Autodesk Inventor part; units mm, degrees
ref_plane "YZ Plane" through (0, 0, 0) normal (1, 0, 0) x (0, 1, 0)
ref_plane "XZ Plane" through (0, 0, 0) normal (0, 1, 0) x (-1, 0, 0)
ref_plane "XY Plane" through (0, 0, 0) normal (0, 0, 1) x (1, 0, 0)
sketch "Sketch1" plane through (0, 0, 0) normal (0, 0, 1) x (1, 0, 0)
  line L0 (0, 0) -> (-15, 0) construction
  circle A0 centre (-15, 0) radius 4
  line L1 (10, 25) -> (0, 25)
  line L2 (0, 25) -> (0, -25)
  line L3 (0, -25) -> (10, -25)
  line L4 (10, -25) -> (10, 25)
  line L5 (0, 0) -> (-15, 0) construction
  line L6 (0, 7) -> (-15, 7)
  line L7 (-15, -7) -> (0, -7)
  arc A1 (0, -7) -> (0, 7) centre (0, 0) ccw
  arc A2 (-15, 7) -> (-15, -7) centre (-15, 0) ccw
  point P0 (-7.5, 0)
  dimension "d0" = 8
  dimension "d1" = 15
  dimension "d2" = 50
  dimension "d3" = 10
  dimension "d4" = 7
extrude "Extrusion1" add sketch "Sketch1" along normal blind 20
sketch "Sketch2" plane through (10, -25, 0) normal (1, 0, 0) x (0, 0, -1)
  line L0 (0, 50) -> (-20, 50) construction
  line L1 (-10, 50) -> (-10, 40) construction
  line L2 (0, 0) -> (-20, 0) construction
  line L3 (-10, 0) -> (-10, 10) construction
  circle A0 centre (-10, 40) radius 2.5
  circle A1 centre (-10, 10) radius 2.5
  point P0 (0, 25)
  dimension "d7" = 5
  dimension "d8" = 10
extrude "Extrusion2" cut sketch "Sketch2" against normal through all
fillet "Fillet1" radius 6 4 edges at (5, 25, 20) (5, 25, 0) (5, -25, 20) (5, -25, 0)
sketch "Sketch3" plane through (10, -19, 0) normal (1, 0, 0) x (0, 0, -1)
  line L0 (-20, 15) -> (-20, 23)
  line L1 (-20, 19) -> (-30, 19) construction
  line L2 (-20, 26) -> (-30, 26)
  line L3 (-30, 12) -> (-20, 12)
  arc A0 (-20, 12) -> (-20, 26) centre (-20, 19) ccw
  arc A1 (-30, 26) -> (-30, 12) centre (-30, 19) ccw
  circle A2 centre (-30, 19) radius 2.5
  point P0 (0, 19)
  point P1 (-25, 19)
  dimension "d12" = 5
  dimension "d13" = 7
  dimension "d14" = 10
extrude "Extrusion3" add sketch "Sketch3" against normal blind 10
properties part number "frame mount 1"
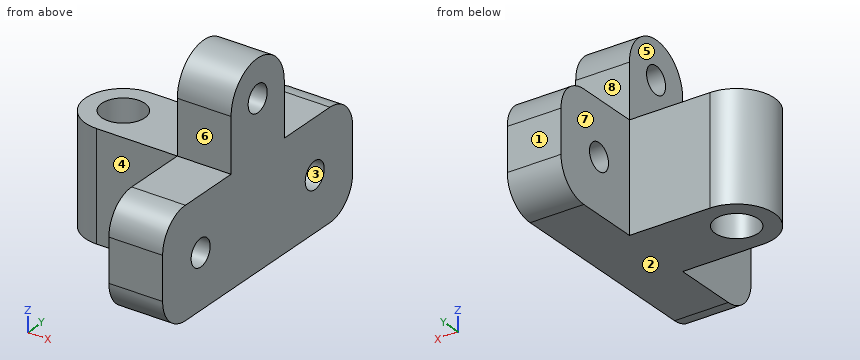
Check sheet for the modelled part. Datum: model origin and axes. Units: mm. Face numbers are marked on the shaded views. A direction names the side the tool comes from. Coordinates: 2 decimals unless noted, no trailing zeros. Write each loop counter-clockwise with the first axis right and the second up, starting at its lowest first coordinate (ties: lowest second). Pieces come first, ordered by that corner, then holes. Notation, with made-up numbers: M -34.5,3.5 L -5.5,3.5 A27 ccw -5.5,19.5 Z; hole C 70,58.25 d6. An arc over 180 degrees is marked long. Use one line per item in the form item = value.
Item 1: Gauge pin test, flat ends, axial feed: pin 1 Ø8 at (x, y) = (-9, -1) entering from +Z; pin 2 Ø7 at (y, z) = (-1, 29) entering from -X; pin 3 Ø14.5 at (y, z) = (-12.5, 8) entering from -X. Record the tip position at first contact, or that the pin passes through.
Answer below:
pin_1 = 20
pin_2 = 0
pin_3 = -19.63
Item 2: Sectioned sample at B-B, the plane z = 10. Record the cut outline in (x, y), and give its area (3 significant figures).
Answer below:
outline = M -15,-7 L 0,-7 L 0,-12.5 L 10,-12.5 L 10,12.5 L 0,12.5 L 0,7 L -15,7 A7 ccw Z; M 0,-25 L 10,-25 L 10,-17.5 L 0,-17.5 Z; M 0,17.5 L 10,17.5 L 10,25 L 0,25 Z; hole C -15,0 d8
area = 637 mm^2
Item 3: Release check for a two-part mould opening along Y. For the marked faces 1, 2 and 3 record: pulls with the +Y half, pulls with the -Y half, needs draft (parallel to the pull), parting line crosses it, or undercut.
Answer below:
face_1 = pulls with the +Y half
face_2 = needs draft
face_3 = undercut
Item 4: Material ranges on L1, parallel to Y at x = 4, z = 10; L2, parallel to Y at x = -15, z = 8.5; L3, parallel to X at y = 2, z = 22.5, recorded low to high. Write a range as from..to.
Answer below:
L1 = -25..-17.5, -12.5..12.5, 17.5..25
L2 = -7..-4, 4..7
L3 = 0..10
Item 5: Sectioned sample at D-D, the plane y = 0. Record the cut outline in (x, z).
Answer below:
outline = M -22,0 L -19,0 L -19,20 L -22,20 Z; M -11,0 L 10,0 L 10,27.5 L 0,27.5 L 0,20 L -11,20 Z; M 0,32.5 L 10,32.5 L 10,37 L 0,37 Z
Item 6: Set-up check for the marked faces 4, 5, 6, 7 and 8: record each of +Z, -Z, +X, -X, +Y, -Y from which the full face is reachable in a straight line by a thin tool's end or side.
Answer below:
face_4 = +Z, -Z, -X, -Y
face_5 = +Z, -X, +Y, -Y
face_6 = +Z, +X, -X, -Y
face_7 = +Z, -Z, -X, +Y
face_8 = +Z, +X, -X, +Y
Item 7: Sectioned sample at A-A, the plane y = -15. Record the cut outline in (x, z), and give its area (3 significant figures).
Answer below:
outline = M 0,0 L 10,0 L 10,7.5 L 0,7.5 Z; M 0,12.5 L 10,12.5 L 10,20 L 0,20 Z
area = 150 mm^2
Item 8: Sectioned sample at C-C, the plane x = 6.5. Record the cut outline in (y, z).
Answer below:
outline = M -25,6 A6 ccw -19,0 L 19,0 A6 ccw 25,6 L 25,14 A6 ccw 19,20 L 7,20 L 7,30 A7 ccw -7,30 L -7,20 L -19,20 A6 ccw -25,14 Z; hole C -15,10 d5; hole C 0,30 d5; hole C 15,10 d5
